The model under review builds one solid part; all positions refer to its coordinate system, in mm. Face numbers are marked on the shaded views. Round coordinates to 2 decimals unless told otherwise and drop trailing zeros. Loops run counter-clockwise (first coordinate to the right, second up) from the corner with the lowest first, then second, coordinate; pieces in that order, holes last. Notation, with made-up numbers: (60, 46) -> (114, 46) arc R20 ccw to (114, 81) -> close; hole circle Ø7 at (76, 71). An arc over 180 degrees is marked (long way). Return JSON: item names as keys, results as strings. Group by question number.
Autodesk Inventor part; units mm, degrees
ref_plane "YZ Plane" through (0, 0, 0) normal (1, 0, 0) x (0, 1, 0)
ref_plane "XZ Plane" through (0, 0, 0) normal (0, 1, 0) x (-1, 0, 0)
ref_plane "XY Plane" through (0, 0, 0) normal (0, 0, 1) x (1, 0, 0)
sketch "Esquisse1" plane through (0, 0, 0) normal (1, 0, 0) x (0, 1, 0)
  circle A0 centre (0, 0) radius 13.8
  dimension "d0" = 27.6
extrude "Extrusion1" add sketch "Esquisse1" along normal blind 8
sketch "Esquisse4" plane through (8, 0, 0) normal (1, 0, 0) x (0, 0, -1)
  circle A0 centre (0, 0) radius 4
  dimension "d13" = 8
extrude "Extrusion4" cut sketch "Esquisse4" against normal blind 4.3
sketch "Esquisse5" plane through (3.7, 0, 0) normal (1, 0, 0) x (0, 0, -1)
  circle A0 centre (0, 0) radius 1.75
  dimension "d16" = 3.5
extrude "Extrusion5" cut sketch "Esquisse5" against normal blind 4.3
fillet "Congé4" radius 1 3 edges at (8, 0, 4) (0, -13.8, 0) (8, -13.8, 0)
properties part number "roue_Impression 3D"
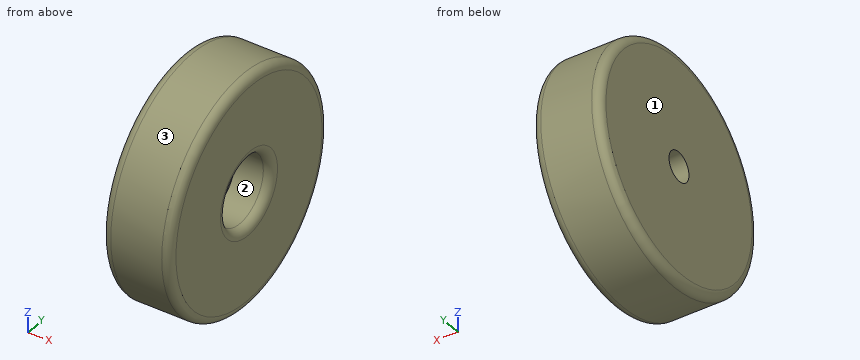
1. For P1, Ø5.5, axis at y = 0, z = 0, coming from the +X side; P2, Ø1.5, axis at x = 6, z = 3, coming from the +Y side; P3, Ø2, axis at x = 1.5, y = 6.5, coming from the -Z side, all flat-tipped, find the tip position at first contact; note any pin that passes through.
2. We need section A-A, the plane y = 0. Write out the cut boundary in (x, z), then the cut area to 3 significant figures.
3. Draft analysis for pull direction Z (two halves, no side actions). For the marked faces 1, 2 and 3, state which applies: pulls with the +Z half, pulls with the -Z half, needs draft (parallel to the pull), parting line crosses it, or undercut.
4. We need section D-D, the plane x = 5.25. Write out the cut boundary in (y, z).
5. Wall thickness on line 1 (Y direction, x = 0.5, z = 1); line 2 (X direction, y = -1, z = -2.25); line 3 (Y direction, x = 3.5, z = -7.5): over which ranges is each line inside the solid? List them lowest first.
6. We need section C-C, the plane x = 2. Write out the cut boundary in (y, z).
Check sheet entries:
{
 "1": {"P1": "stops at x = 3.7", "P2": "stops at y = 13.62", "P3": "stops at z = -12.66"},
 "2": {"outline": "(0, -12.8) arc R1 ccw to (1, -13.8) -> (7, -13.8) arc R1 ccw to (8, -12.8) -> (8, -5) arc R1 ccw to (7, -4) -> (3.7, -4) -> (3.7, -1.75) -> (0, -1.75) -> close; (0, 1.75) -> (3.7, 1.75) -> (3.7, 4) -> (7, 4) arc R1 ccw to (8, 5) -> (8, 12.8) arc R1 ccw to (7, 13.8) -> (1, 13.8) arc R1 ccw to (0, 12.8) -> close", "area": "172 mm²"},
 "3": {"face 1": "needs draft", "face 2": "undercut", "face 3": "parting line crosses it"},
 "4": {"outline": "circle Ø27.6 at (0, 0); hole circle Ø8 at (0, 0)"},
 "5": {"line 1": "y = -13.63 to -1.44, 1.44 to 13.63", "line 2": "x = 0 to 3.7", "line 3": "y = -11.58 to 11.58"},
 "6": {"outline": "circle Ø27.6 at (0, 0); hole circle Ø3.5 at (0, 0)"}
}
